Answer from the drawing. Dimensions are ordinates in mm from the lowest x, y and z of the part. A direction names the side the tool comes from. Coordinates: 2 decimals unless noted, no trailing zeros. Order: outer loops, then holes, each group sorted by start corner. A loop starts at its lowest first (then second) coordinate and runs counter-clockwise, first axis right, second up. Notation, with made-up numbers: M 46.25,-5.75 L 98.25,-5.75 A35 cw 98.25,32.25 Z; hole C 6,78.5 d6. An arc over 180 degrees is marked long. Write each question's results on one line, items separated by ' | '.
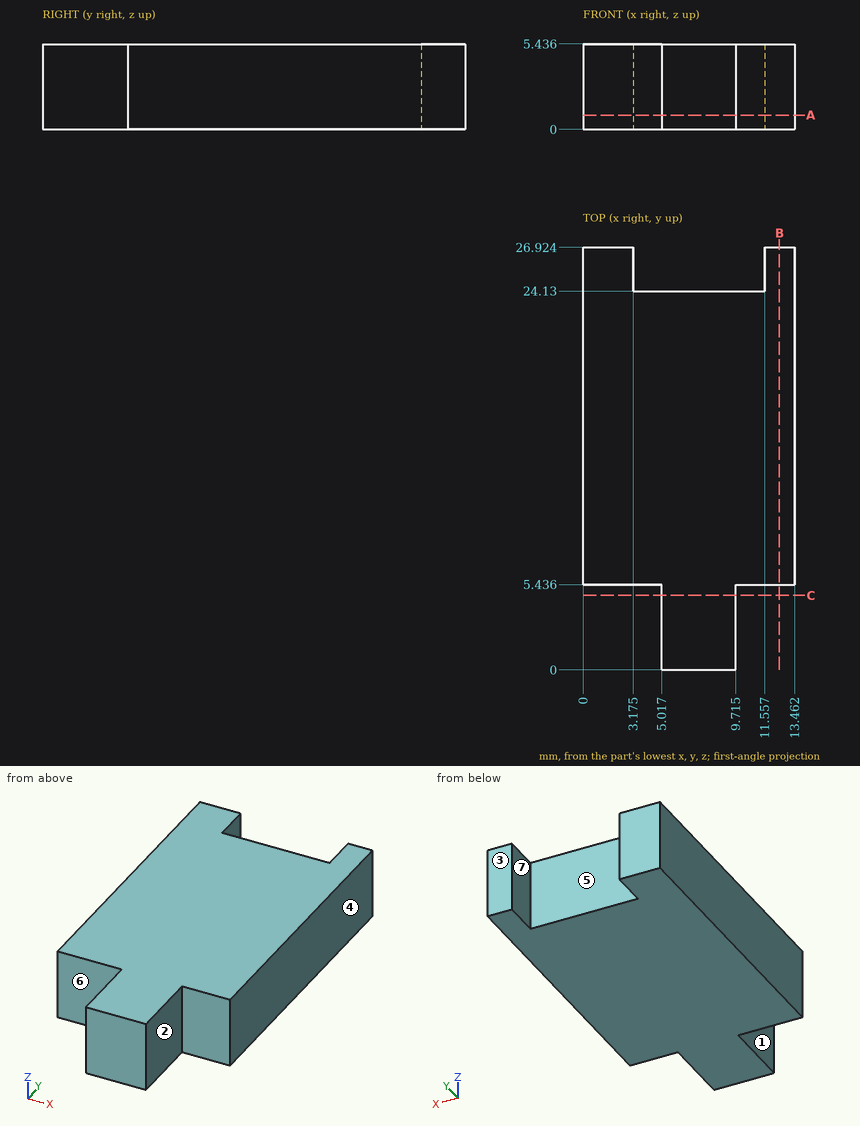
(1) For the marked faces 1, 2 and 3, determine the directions among +Z, -Z, +X, -X, +Y, -Y from which every point of the face is accessible in a straight line to the end or side of a thin tool.
Conclusion:
face 1: +Z, -Z, -X, -Y | face 2: +Z, -Z, +X, -Y | face 3: +Z, -Z, +X, -X, +Y
(2) Given pin 1 (1.5 mm diameter, centred on x = 3, z = 3, fed in from -Y); pin 2 (1.6 mm diameter, centred on y = 2, z = 2.5, fed in from +X) (1 decimal); pin 3 (2.5 mm diameter, centred on x = 6, z = 3, fed in from +Y), each flat-ended and moving along its own axis, determine where each tip first touches the part or whether it passes through.
Conclusion:
pin 1: y = 5.44 | pin 2: x = 9.7 | pin 3: y = 24.13
(3) The part is cut by section B-B, the plane x = 12.5. Write down the section's boundary in (y, z) (1 decimal).
Conclusion:
outline: M 5.4,0 L 26.9,0 L 26.9,5.4 L 5.4,5.4 Z
(4) The mould has two halves that part along X. Classify the marked faces 4, 5, 6 and 7: pulls with the +X half, pulls with the -X half, needs draft (parallel to the pull), parting line crosses it, or undercut.
Conclusion:
face 4: pulls with the +X half | face 5: undercut | face 6: needs draft | face 7: undercut
(5) The part is cut by section A-A, the plane z = 0.9. Write down the section's boundary in (x, y) (1 decimal), then the cut area to 3 significant figures.
Conclusion:
outline: M 0,5.4 L 5,5.4 L 5,0 L 9.7,0 L 9.7,5.4 L 13.5,5.4 L 13.5,26.9 L 11.6,26.9 L 11.6,24.1 L 3.2,24.1 L 3.2,26.9 L 0,26.9 Z | area: 291 mm²
(6) Straight lines are drawn through the part: line 1 (X direction, y = 4, z = 2.5) (1 decimal); line 2 (Y direction, x = 6.25, z = 4.6); line 3 (Y direction, x = 0.75, z = 3.05) (1 decimal). For each, find the intervals that lie inside material, in ascending order.
Conclusion:
line 1: 5 to 9.7 | line 2: 0 to 24.13 | line 3: 5.4 to 26.9
(7) The part is cut by section C-C, the plane y = 4.75. Write down the section's boundary in (x, z) (1 decimal).
Conclusion:
outline: M 5,0 L 9.7,0 L 9.7,5.4 L 5,5.4 Z
